Input: dimensioned drawing with shaded views. Units: mm. Origin: part minimum x, y, z. Coordinates: 2 decimals unless noted, no trailing zeros. Order: outer loops, then holes, each group sorted by start corner. A loop starts at its lowest first (then second) coordinate and runs counter-clockwise, first axis right, second up. Notation, with made-up numbers: (-28, 86.25) -> (-12, 86.25) arc R34 ccw to (-12, 121.25) -> close; hole circle Ø6 at (-40, 88). An arc over 180 degrees is marked (long way). Answer in a Markdown table with one row per item. Add a question column.
1) Section query D-D on y = 17.5. Return the cut outline in (x, z), then the cut area to 3 significant figures.
2) Section query B-B on z = 1.6. Return the cut outline in (x, y), then the cut area to 3 significant figures.
3) Ray query, line 1 (X direction, y = 19.5, z = 1.75); line 2 (X direction, y = 20, z = 2.65); line 3 (X direction, y = 11.5, z = 1.8). Return the intervals inside material, ascending. Write a range as from..to.
4) Contact query for flat-ended pins moving along their axis: P1, Ø1.5, axis at x = 61.5, z = 2, coming from the -Y side; P2, Ø1.5, axis at x = 15.5, z = 1, coming from the -Y side; P3, Ø0.9, axis at y = 30, z = 2, coming from the +X side. Output: stop coordinate, or through.
5) Section query C-C on y = 6.5. Return the cut outline in (x, z).
6) Section query A-A on y = 31. Return the cut outline in (x, z).
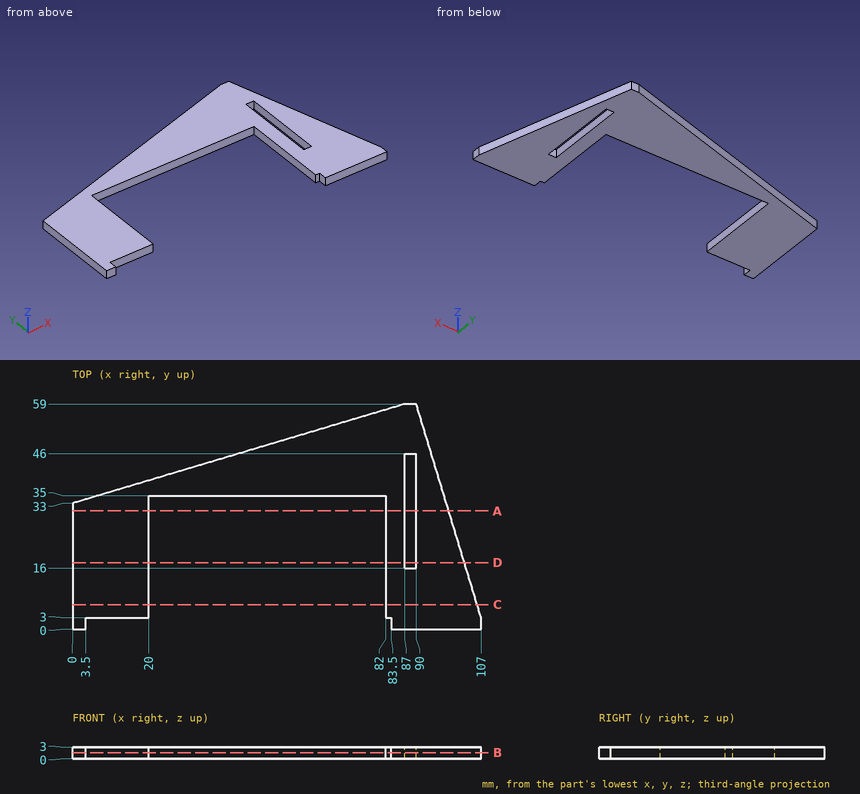
Result:
| question | item | result |
|---|---|---|
| 1 | outline | (0, 0) -> (20, 0) -> (20, 3) -> (0, 3) -> close; (82, 0) -> (87, 0) -> (87, 3) -> (82, 3) -> close; (90, 0) -> (102.6, 0) -> (102.6, 3) -> (90, 3) -> close |
| 1 | area | 113 mm2 |
| 2 | outline | (0, 0) -> (3.5, 0) -> (3.5, 3) -> (20, 3) -> (20, 35) -> (82, 35) -> (82, 3) -> (83.5, 3) -> (83.5, 0) -> (107, 0) -> (107, 3) -> (90, 59) -> (87, 59) -> (0, 33) -> close; hole (87, 16) -> (90, 16) -> (90, 46) -> (87, 46) -> close |
| 2 | area | 2,390 mm2 |
| 3 | line 1 | 0..20, 82..87, 90..101.99 |
| 3 | line 2 | 0..20, 82..87, 90..101.84 |
| 3 | line 3 | 0..20, 82..104.42 |
| 4 | P1 | y = 35 |
| 4 | P2 | y = 3 |
| 4 | P3 | x = 98.94 |
| 5 | outline | (0, 0) -> (20, 0) -> (20, 3) -> (0, 3) -> close; (82, 0) -> (105.94, 0) -> (105.94, 3) -> (82, 3) -> close |
| 6 | outline | (0, 0) -> (20, 0) -> (20, 3) -> (0, 3) -> close; (82, 0) -> (87, 0) -> (87, 3) -> (82, 3) -> close; (90, 0) -> (98.5, 0) -> (98.5, 3) -> (90, 3) -> close |
